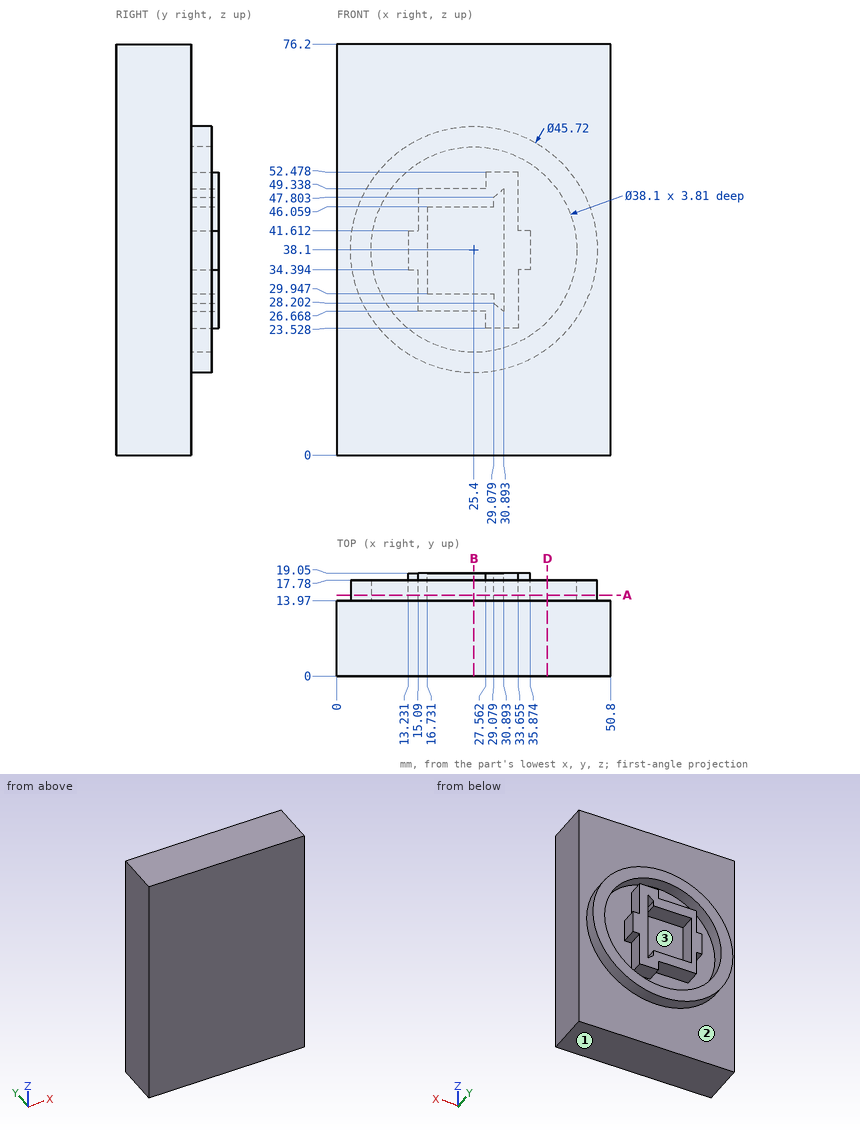
Source: three-view drawing plus pictorial views. Frame: mm from the lowest corner of the part. Round coordinates to 2 decimals unless told otherwise and drop trailing zeros. Loops run counter-clockwise (first coordinate to the right, second up) from the corner with the lowest first, then second, coordinate; pieces in that order, holes last.
Q1. Section B-B on x = 25.4. Return loops of the section in (y, z), plus the area to 3 significant figures.
Q2. Section D-D on x = 39. Return loops of the section in (y, z) (1 decimal), plus the area to 3 significant figures.
Q3. Pin query (flat end, axial travel): P1, Ø2.5, axis at y = 15.5, z = 41.5, coming from the +X side; P2, Ø2.5, axis at x = 21, y = 17, coming from the +Z side; P3, Ø4, axis at x = 11.5, z = 37.5, coming from the +Y side; P4, Ø1.8, axis at x = 35, y = 17.5, coming from the +Z side. Return the tip coordinate at first contact, or that it passes through.
Q4. Pull-direction query (Z, two-part tool) for the marked faces 1, 2 and 3; classes: released by +Z, released by -Z, zero draft, split by the parting line, or undercut.
Q5. Section A-A on y = 15. State how many separate pieces and enclosed holes the cut face has.
Q6. Material intervals for L1, parallel to Z at x = 25.4, y = 14.8; L2, parallel to Y at x = 48, z = 58.5; L3, parallel to Y at x = 4, z = 41.5, sorted ascending.
Evaluation:
1. outline: (0, 0) - (13.97, 0) - (13.97, 15.24) - (17.78, 15.24) - (17.78, 19.05) - (13.97, 19.05) - (13.97, 26.67) - (19.05, 26.67) - (19.05, 29.95) - (13.97, 29.95) - (13.97, 46.06) - (19.05, 46.06) - (19.05, 49.34) - (13.97, 49.34) - (13.97, 57.15) - (17.78, 57.15) - (17.78, 60.96) - (13.97, 60.96) - (13.97, 76.2) - (0, 76.2) - close
1. area: 1,130 mm2
2. outline: (0, 0) - (14, 0) - (14, 19.7) - (17.8, 19.7) - (17.8, 24.8) - (14, 24.8) - (14, 51.4) - (17.8, 51.4) - (17.8, 56.5) - (14, 56.5) - (14, 76.2) - (0, 76.2) - close
2. area: 1,100 mm2
3. P1: stops at x = 48.16
3. P2: stops at z = 60.74
3. P3: stops at y = 19.05
3. P4: stops at z = 59.24
4. face 1: released by -Z
4. face 2: zero draft
4. face 3: undercut
5. separate pieces: 2
5. enclosed holes: 2
6. L1: z = 15.24 to 19.05, 26.67 to 29.95, 46.06 to 49.34, 57.15 to 60.96
6. L2: y = 0 to 13.97
6. L3: y = 0 to 17.78
